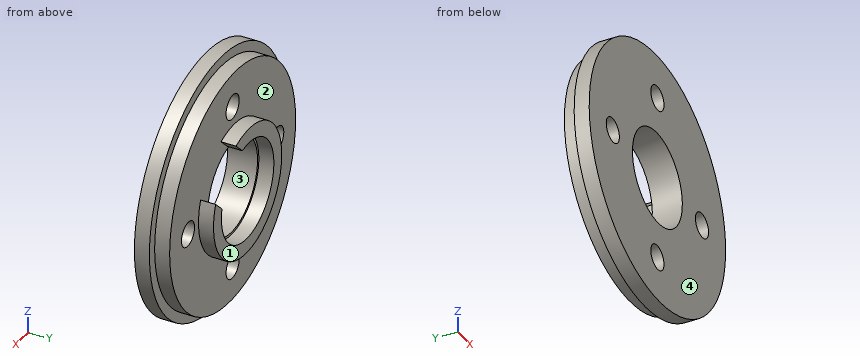
from build123d import *

# Parameters (mm, degrees)
SKETCH1_R           = 13
BOSS_EXTRUDE1_DEPTH = 1.5
SKETCH2_R           = 12
BOSS_EXTRUDE2_DEPTH = 1.5
SKETCH3_R           = 6.5
BOSS_EXTRUDE3_DEPTH = 1.5
SKETCH4_R           = 1.25
CUT_EXTRUDE1_DEPTH  = 11.5
SKETCH5_R           = 4.75
CUT_EXTRUDE2_DEPTH  = 11.5
SKETCH6_R           = 5
CUT_EXTRUDE3_DEPTH  = 1.5
CUT_EXTRUDE4_DEPTH  = 1.5


with BuildPart() as part:
    # Sketch1 → Boss-Extrude1 (new body)
    with BuildSketch(Plane(origin=(0, 0, 0), x_dir=(1, 0, 0), z_dir=(0, 1, 0))):
        with Locations(Location((0, 0, 0), (0, 0, 270))):
            Circle(SKETCH1_R)
    extrude(amount=BOSS_EXTRUDE1_DEPTH)

    # Sketch2 → Boss-Extrude2 (add)
    with BuildSketch(Plane(origin=(0, 1.5, 0), x_dir=(1, 0, 0), z_dir=(0, 1, 0))):
        with Locations(Location((0, 0, 0), (0, 0, 270))):
            Circle(SKETCH2_R)
    extrude(amount=BOSS_EXTRUDE2_DEPTH)

    # Sketch3 → Boss-Extrude3 (add)
    with BuildSketch(Plane(origin=(0, 3, 0), x_dir=(1, 0, 0), z_dir=(0, 1, 0))):
        with Locations(Location((0, 0, 0), (0, 0, 270))):
            Circle(SKETCH3_R)
    extrude(amount=BOSS_EXTRUDE3_DEPTH)

    # Sketch4 → Cut-Extrude1 (cut)
    with BuildSketch(Plane(origin=(0, 3, 0), x_dir=(1, 0, 0), z_dir=(0, 1, 0))):
        with Locations(Location((-8.5, 0, 0), (0, 0, 270))):
            Circle(SKETCH4_R)
        with Locations(Location((0, 8.5, 0), (0, 0, 270))):
            Circle(SKETCH4_R)
        with Locations(Location((8.5, 0, 0), (0, 0, 270))):
            Circle(SKETCH4_R)
        with Locations(Location((0, -8.5, 0), (0, 0, 270))):
            Circle(SKETCH4_R)
    extrude(amount=-CUT_EXTRUDE1_DEPTH, mode=Mode.SUBTRACT)

    # Sketch5 → Cut-Extrude2 (cut)
    with BuildSketch(Plane(origin=(0, 4.5, 0), x_dir=(1, 0, 0), z_dir=(0, 1, 0))):
        with Locations(Location((0, 0, 0), (0, 0, 270))):
            Circle(SKETCH5_R)
    extrude(amount=-CUT_EXTRUDE2_DEPTH, mode=Mode.SUBTRACT)

    # Sketch6 → Cut-Extrude3 (cut)
    with BuildSketch(Plane(origin=(0, 4.5, 0), x_dir=(1, 0, 0), z_dir=(0, 1, 0))):
        with Locations(Location((0, 0, 0), (0, 0, 270))):
            Circle(SKETCH6_R)
    extrude(amount=-CUT_EXTRUDE3_DEPTH, mode=Mode.SUBTRACT)

    # Sketch7 → Cut-Extrude4 (cut)
    with BuildSketch(Plane(origin=(0, 4.5, 0), x_dir=(1, 0, 0), z_dir=(0, 1, 0))):
        Polygon((0.767606776, -4.656694072), (4.656694072, -0.767606776), (9.347013617, -5.457926321), (5.457926321, -9.347013617), align=None)
    extrude(amount=-CUT_EXTRUDE4_DEPTH, mode=Mode.SUBTRACT)


solid = part.part
CAD build for the part. Positions are in the model's coordinates, mm. Face numbers are marked on the shaded views. A direction names the side the tool comes from. Round coordinates to 2 decimals unless told otherwise and drop trailing zeros. Order: outer loops, then holes, each group sorted by start corner. A loop starts at its lowest first (then second) coordinate and runs counter-clockwise, first axis right, second up. Notation, with made-up numbers: (64.25, -33.5) - (72.25, -33.5) arc R33 cw to (72.25, -1.5) - close; hole circle Ø8 at (33.5, 89.25). An arc over 180 degrees is marked (long way). Return JSON: item names as keys, results as strings.
(1) Cut at B-B (z = 0.5). Give the cut face in (x, y).
Answer key:
{"outline": "(-12.99, 0) - (-9.65, 0) - (-9.65, 3) - (-11.99, 3) - (-11.99, 1.5) - (-12.99, 1.5) - close; (-7.35, 0) - (-4.72, 0) - (-4.72, 3) - (-4.97, 3) - (-4.97, 4.5) - (-6.48, 4.5) - (-6.48, 3) - (-7.35, 3) - close; (4.72, 0) - (7.35, 0) - (7.35, 3) - (6.48, 3) - (6.48, 4.5) - (4.97, 4.5) - (4.97, 3) - (4.72, 3) - close; (9.65, 0) - (12.99, 0) - (12.99, 1.5) - (11.99, 1.5) - (11.99, 3) - (9.65, 3) - close"}
(2) Pin check, flat tips, straight feed: pin 1 Ø3 at (x, z) = (0, 8.5) entering from +Y; pin 2 Ø1.5 at (x, y) = (9.5, 2.5) entering from -Z; pin 3 Ø2 at (x, z) = (0, -8.5) entering from -Y; pin 4 Ø2 at (x, y) = (2, 3.5) entering from +Z. Stop position of each tip, or through.
Answer key:
{"pin 1": "stops at y = 3", "pin 2": "stops at z = -8.21", "pin 3": "passes through", "pin 4": "stops at z = 11.95"}
(3) Cut at D-D (z = -2.75). Give the cut face in (x, y).
Answer key:
{"outline": "(-12.71, 0) - (-3.87, 0) - (-3.87, 3) - (-4.18, 3) - (-4.18, 4.5) - (-5.89, 4.5) - (-5.89, 3) - (-11.68, 3) - (-11.68, 1.5) - (-12.71, 1.5) - close; (3.87, 0) - (12.71, 0) - (12.71, 1.5) - (11.68, 1.5) - (11.68, 3) - (5.89, 3) - (5.89, 4.5) - (4.18, 4.5) - (4.18, 3) - (3.87, 3) - close"}
(4) Tool access for the marked faces 1 and 2: list every direction of +Z, -Z, +X, -X, +Y, -Y with a clear straight run to the whole face (end or side of a thin tool).
Answer key:
{"face 1": "+Z, -Z, +X, -X, +Y", "face 2": "+Y"}
(5) Cut at C-C (x = 8.5). Give the cut face in (y, z), then the cut area to 3 significant figures.
Answer key:
{"outline": "(0, -9.84) - (1.5, -9.84) - (1.5, -8.47) - (3, -8.47) - (3, -1.25) - (0, -1.25) - close; (0, 1.25) - (3, 1.25) - (3, 8.47) - (1.5, 8.47) - (1.5, 9.84) - (0, 9.84) - close", "area": "47.4 mm^2"}
(6) Wall check: probe 1 along X at (y, z) = (0.9, 0); probe 2 along Z at (x, y) = (0, 3.9); probe 3 along Y at (x, z) = (5.75, -3.5). Give the ranges that are in metal, low to high. Write a range as from..to.
Answer key:
{"probe 1": "x = -13..-9.75, -7.25..-4.75, 4.75..7.25, 9.75..13", "probe 2": "z = -6.5..-5, 5..6.5", "probe 3": "y = 0..3"}
(7) Pull direction X, two halves, no side cores. Call the marked faces 3 and 4: +X half, -X half, draft (parallel to the pull), parting line (faces both ways), or undercut.
Answer key:
{"face 3": "undercut", "face 4": "draft"}
(8) Cut at A-A (y = 0.5). Give the cut face in (x, z).
Answer key:
{"outline": "circle Ø26 at (0, 0); hole circle Ø2.5 at (-8.5, 0); hole circle Ø9.5 at (0, 0); hole circle Ø2.5 at (0, -8.5); hole circle Ø2.5 at (0, 8.5); hole circle Ø2.5 at (8.5, 0)"}
